Study the drawing (mm; zero at the part's minimum x, y, z) and answer. A direction names the side the tool comes from. Coordinates: 2 decimals unless noted, no trailing zeros. Loops run counter-clockwise (first coordinate to the right, second up) from the corner with the lowest first, then second, coordinate; pieces in that order, holes last. Notation, with made-up numbers: (74, -4.75) -> (97, -4.75) arc R22 cw to (97, 11.25) -> close; hole circle Ø5 at (14.25, 2.25). An arc over 180 degrees is marked (long way). Answer as CSV lines item,"result".
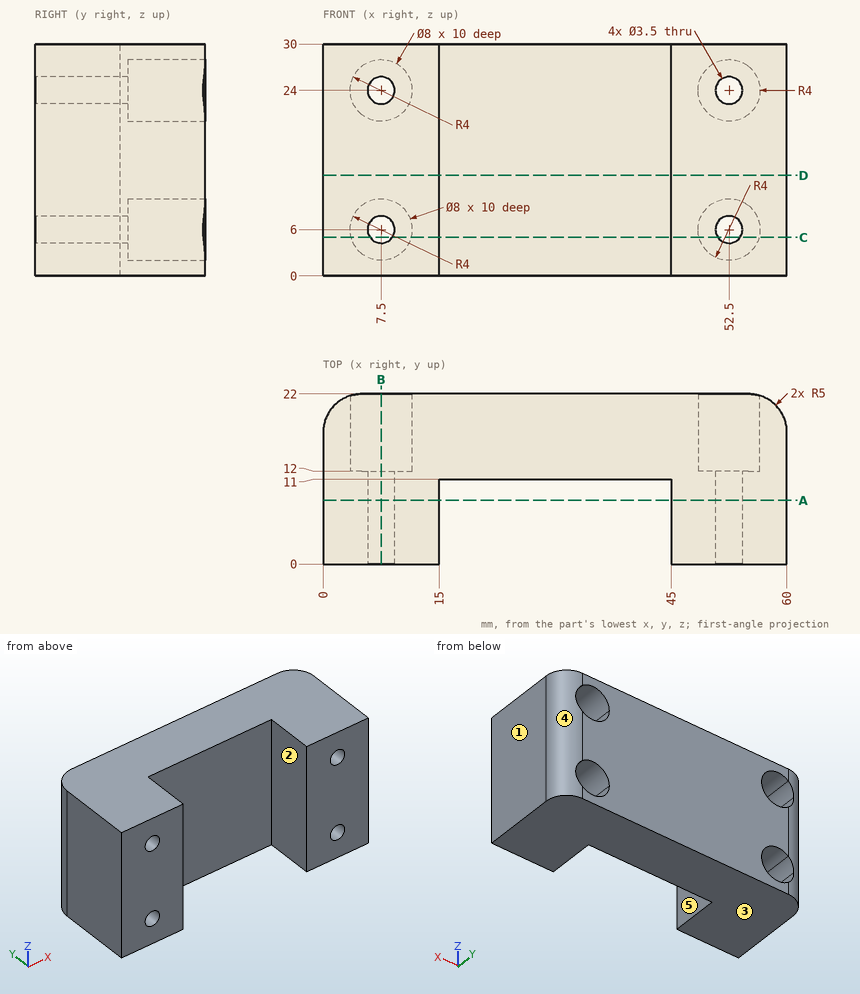
Q1. Find the intervals of material crossed by probe 1 along Z at (x, y) = (7.5, 19.5); probe 2 along Z at (x, y) = (50, 19.75); probe 3 along X at (y, z) = (13.5, 23.5), in increasing order. Write a range as [from, to].
Results:
probe 1,"z = [0, 2], [10, 20], [28, 30]"
probe 2,"z = [0, 2.88], [9.12, 20.88], [27.12, 30]"
probe 3,"x = [0, 3.53], [11.47, 48.53], [56.47, 60]"
Q2. For the marked faces 1 and 2, determine the directions among +Z, -Z, +X, -X, +Y, -Y from which every point of the face is accessible in a straight line to the end or side of a thin tool.
Results:
face 1,"+Z, -Z, +X, +Y, -Y"
face 2,"+Z, -Z, -Y"
Q3. A cutting plane is placed at A-A, the plane y = 8.25. Write down the section's boundary in (x, z), and give its area (3 significant figures).
Results:
outline,"(0, 0) -> (15, 0) -> (15, 30) -> (0, 30) -> close; (45, 0) -> (60, 0) -> (60, 30) -> (45, 30) -> close; hole circle Ø3.5 at (7.5, 6); hole circle Ø3.5 at (7.5, 24); hole circle Ø3.5 at (52.5, 6); hole circle Ø3.5 at (52.5, 24)"
area,"862 mm²"
Q4. A cutting plane is placed at B-B, the plane x = 7.5. Write down the section's boundary in (y, z).
Results:
outline,"(0, 0) -> (22, 0) -> (22, 2) -> (12, 2) -> (12, 4.25) -> (0, 4.25) -> close; (0, 7.75) -> (12, 7.75) -> (12, 10) -> (22, 10) -> (22, 20) -> (12, 20) -> (12, 22.25) -> (0, 22.25) -> close; (0, 25.75) -> (12, 25.75) -> (12, 28) -> (22, 28) -> (22, 30) -> (0, 30) -> close"
Q5. A cutting plane is placed at C-C, the plane z = 5. Write down the section's boundary in (x, y).
Results:
outline,"(0, 0) -> (6.06, 0) -> (6.06, 12) -> (3.63, 12) -> (3.63, 21.81) arc R5 ccw to (0, 17) -> close; (8.94, 0) -> (15, 0) -> (15, 11) -> (45, 11) -> (45, 0) -> (51.06, 0) -> (51.06, 12) -> (48.63, 12) -> (48.63, 22) -> (11.37, 22) -> (11.37, 12) -> (8.94, 12) -> close; (53.94, 0) -> (60, 0) -> (60, 17) arc R5 ccw to (56.37, 21.81) -> (56.37, 12) -> (53.94, 12) -> close"
Q6. Given pin 1 Ø4 at (x, z) = (7.5, 6) entering from +Y; pin 2 Ø2 at (y, z) = (20, 11.5) entering from -X; pin 3 Ø9 at (x, z) = (53.5, 22.5) entering from +Y, each flat-ended and moving along its own axis, determine where each tip first touches the part or whether it passes through.
Results:
pin 1,"stops at y = 12"
pin 2,"stops at x = 0.42"
pin 3,"stops at y = 22"
Q7. A cutting plane is placed at D-D, the plane z = 13. Write down the section's boundary in (x, y).
Results:
outline,"(0, 0) -> (15, 0) -> (15, 11) -> (45, 11) -> (45, 0) -> (60, 0) -> (60, 17) arc R5 ccw to (55, 22) -> (5, 22) arc R5 ccw to (0, 17) -> close"
Q8. For a pull along X with two mould halves and no side action, classify the marked faces 3, 4 and 5 as pulls with the +X half, pulls with the -X half, needs draft (parallel to the pull), parting line crosses it, or undercut.
Results:
face 3,"needs draft"
face 4,"pulls with the +X half"
face 5,"undercut"
